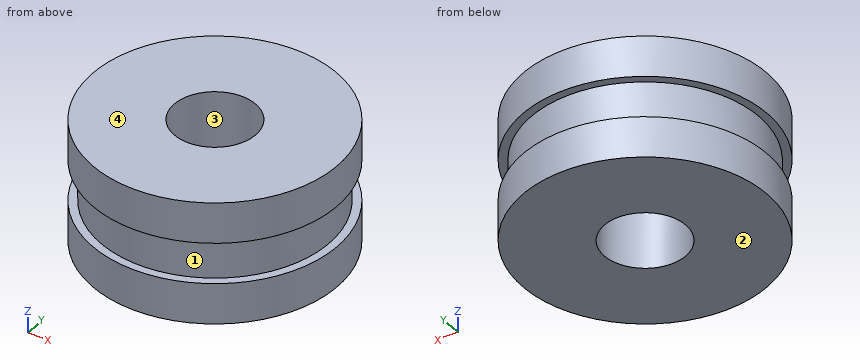
from build123d import *

# Parameters (mm, degrees)
EXTRUDE_1_DEPTH          = 1.5
EXTRUDE_1_DEPTH_BACK     = 1.5
SKETCH_1_R               = 3
SKETCH_1_R_2             = 1
CUT_EXTRUDE_1_DEPTH      = 0.5
CUT_EXTRUDE_1_DEPTH_BACK = 0.5
SKETCH_2_R               = 3
SKETCH_2_R_2             = 2.8


with BuildPart() as part:
    # 草图1 → 凸台-拉伸1 (new, two sides: drawn at the far end of the back side and taken through both)
    with BuildSketch(Plane.XY.offset(-EXTRUDE_1_DEPTH_BACK)):
        Circle(SKETCH_1_R)
        Circle(SKETCH_1_R_2, mode=Mode.SUBTRACT)
    extrude(amount=EXTRUDE_1_DEPTH + EXTRUDE_1_DEPTH_BACK)

    # 草图2 → 切除-拉伸1 (cut, two sides: drawn at the far end of the back side and taken through both)
    with BuildSketch(Plane.XY.offset(-CUT_EXTRUDE_1_DEPTH_BACK)):
        Circle(SKETCH_2_R)
        Circle(SKETCH_2_R_2, mode=Mode.SUBTRACT)
    extrude(amount=CUT_EXTRUDE_1_DEPTH + CUT_EXTRUDE_1_DEPTH_BACK, mode=Mode.SUBTRACT)


solid = part.part
CAD build for the part. Positions are in the model's coordinates, mm. Face numbers are marked on the shaded views. Round coordinates to 2 decimals unless told otherwise and drop trailing zeros. Order: outer loops, then holes, each group sorted by start corner. A loop starts at its lowest first (then second) coordinate and runs counter-clockwise, first axis right, second up. Notation, with made-up numbers: (46.5, -3.5) -> (51.5, -3.5) arc R31 ccw to (51.5, 31.5) -> close; hole circle Ø3 at (-4, 52). An arc over 180 degrees is marked (long way). Write item = value, one per line. Start each with the question number.
(1) Cut at A-A, the plane x = 0. List the corners of the cut face in (y, z), then the cut area to 3 significant figures.
(2) Probe line 1 (Z direction, x = -1.65, y = -2.3); line 2 (Y direction, x = 0, z = -0.65); line 3 (Y direction, x = 0, z = 0.4). List the from-to ranges inside material, lowest first. Write a range as [from, to].
(3) Pull direction Z, two halves, no side cores. Call the marked faces 1, 2, 3 and 4: released by +Z, released by -Z, zero draft, split by the parting line, or undercut.
(4) Cut at D-D, the plane z = 0.8. List the corners of the cut face in (x, y), then the cut area to 3 significant figures.
(5) Cut at C-C, the plane y = 1.7. List the corners of the cut face in (x, z).
(6) Pin check, flat tips, straight feed: P1, Ø1, axis at y = -1, z = -0.5, coming from the -X side; P2, Ø1.6, axis at x = 0, y = 0, coming from the -Z side. Stop position of each tip, or through.
Model answer:
q1.outline = (-3, -1.5) -> (-1, -1.5) -> (-1, 1.5) -> (-3, 1.5) -> (-3, 0.5) -> (-2.8, 0.5) -> (-2.8, -0.5) -> (-3, -0.5) -> close; (1, -1.5) -> (3, -1.5) -> (3, -0.5) -> (2.8, -0.5) -> (2.8, 0.5) -> (3, 0.5) -> (3, 1.5) -> (1, 1.5) -> close
q1.area = 11.6 mm2
q2.line_1 = [-1.5, -0.5], [0.5, 1.5]
q2.line_2 = [-3, -1], [1, 3]
q2.line_3 = [-2.8, -1], [1, 2.8]
q3.face_1 = undercut
q3.face_2 = released by -Z
q3.face_3 = zero draft
q3.face_4 = released by +Z
q4.outline = circle Ø6 at (0, 0); hole circle Ø2 at (0, 0)
q4.area = 25.1 mm2
q5.outline = (-2.47, -1.5) -> (2.47, -1.5) -> (2.47, -0.5) -> (2.22, -0.5) -> (2.22, 0.5) -> (2.47, 0.5) -> (2.47, 1.5) -> (-2.47, 1.5) -> (-2.47, 0.5) -> (-2.22, 0.5) -> (-2.22, -0.5) -> (-2.47, -0.5) -> close
q6.P1 = -2.96
q6.P2 = through
